```python
from build123d import *

# Parameters (mm, degrees)
SKETCH1_R           = 3
BOSS_EXTRUDE1_DEPTH = 25
SKETCH2_R           = 5
SKETCH2_R_2         = 3
BOSS_EXTRUDE2_DEPTH = 6
FILLET1_R           = 0.3
FILLET2_R           = 0.25


with BuildPart() as part:
    # Sketch1 → Boss-Extrude1 (new body)
    with BuildSketch(Plane(origin=(0, 0, 0), x_dir=(1, 0, 0), z_dir=(0, 1, 0))):
        Circle(SKETCH1_R)
    extrude(amount=BOSS_EXTRUDE1_DEPTH)

    # Sketch2 → Boss-Extrude2 (add)
    with BuildSketch(Plane(origin=(0, 25, 0), x_dir=(1, 0, 0), z_dir=(0, 1, 0))):
        Circle(SKETCH2_R)
        Circle(SKETCH2_R_2, mode=Mode.SUBTRACT)
        Circle(SKETCH2_R_2)
        Polygon((1.913417162, -1.913417162), (2.705980501, 0), (1.913417162, 1.913417162), (0, 2.705980501), (-1.913417162, 1.913417162), (-2.705980501, 0), (-1.913417162, -1.913417162), (0, -2.705980501), align=None, mode=Mode.SUBTRACT)
    extrude(amount=BOSS_EXTRUDE2_DEPTH)

    # Fillet1
    fillet1_edges = [part.edges().sort_by_distance(p)[0] for p in [
        (-5, 31, 0),
    ]]
    fillet(fillet1_edges, radius=FILLET1_R)

    # Fillet2
    fillet2_edges = [part.edges().sort_by_distance(p)[0] for p in [
        (-3, 25, 0),
    ]]
    fillet(fillet2_edges, radius=FILLET2_R)


solid = part.part
```
Design review of the part built by this model. Coordinates are the model's own, in mm. A direction names the side the tool comes from. Coordinates: 2 decimals unless noted, no trailing zeros. Loops run counter-clockwise (first coordinate to the right, second up) from the corner with the lowest first, then second, coordinate; pieces in that order, holes last. Notation, with made-up numbers: (35.25, 35) -> (51.25, 35) arc R19 ccw to (51.25, 68) -> close; hole circle Ø11 at (40, 35.25). An arc over 180 degrees is marked (long way). Answer as a JSON object with one key per item and string values.
Q1. Tool access review of faces 4 (the flat face through (1, 25, 3.3)), 5 (the flat face through (0.943, 27.958, 2.315)), 6 (the flat face through (0, 0, 0)): name each direction out of +Z, -Z, +X, -X, +Y, -Y from which nothing blocks a thin tool from reaching the whole face with its end or side.
Answer block:
{"face 4": "-Y", "face 5": "+Y", "face 6": "+Z, -Z, +X, -X, -Y"}
Q2. The part is to be moulded in two halves that separate along Z. For faces 1 (the flat face through (2.02, 31, 2.02)), 2 (the cylindrical face through (-3, 12, 0)), 3 (the flat face through (-0.97, 27.958, 2.304)), say which applies: +Z half, -Z half, draft (parallel to the pull), parting line (faces both ways), or undercut.
Answer block:
{"face 1": "draft", "face 2": "parting line", "face 3": "undercut"}
Q3. To check wall thickness, follow L1, parallel to Y at x = 2.75, z = -3; L2, parallel to Y at x = -2, z = 1; L3, parallel to X at y = 30.5, z = 1.25. State the ranges of each line that lie inside material, in increasing order.
Answer block:
{"L1": "y = 25 to 31", "L2": "y = 0 to 25", "L3": "x = -4.84 to -2.19, 2.19 to 4.84"}
Q4. Take a section at A-A on y = 8. Give the boundary of the cut face in (x, z).
Answer block:
{"outline": "circle Ø6 at (0, 0)"}
Q5. Clearance check with flat-ended pins moving along their axes: pin 1 Ø3 at (y, z) = (14.5, 0) entering from -X; pin 2 Ø1.5 at (y, z) = (4, -1) entering from +X; pin 3 Ø1.5 at (x, z) = (-3.5, 2.5) entering from -Y. State where each tip first meets the part, or that it passes through.
Answer block:
{"pin 1": "stops at x = -3", "pin 2": "stops at x = 2.99", "pin 3": "stops at y = 25"}
